Source: three-view drawing plus pictorial views. Frame: mm from the lowest corner of the part. A direction names the side the tool comes from. Give positions to 0.01 mm unless a question says otherwise; leave off trailing zeros. Write each loop counter-clockwise with the first axis right and the second up, starting at its lowest first coordinate (ties: lowest second). Pieces come first, ordered by that corner, then holes. Notation, with made-up numbers: M 48.5,28.5 L 72.5,28.5 A16 cw 72.5,57.5 Z; hole C 59.5,-28.75 d4. An arc over 180 degrees is marked long. Return JSON: item names as keys, results as strings.
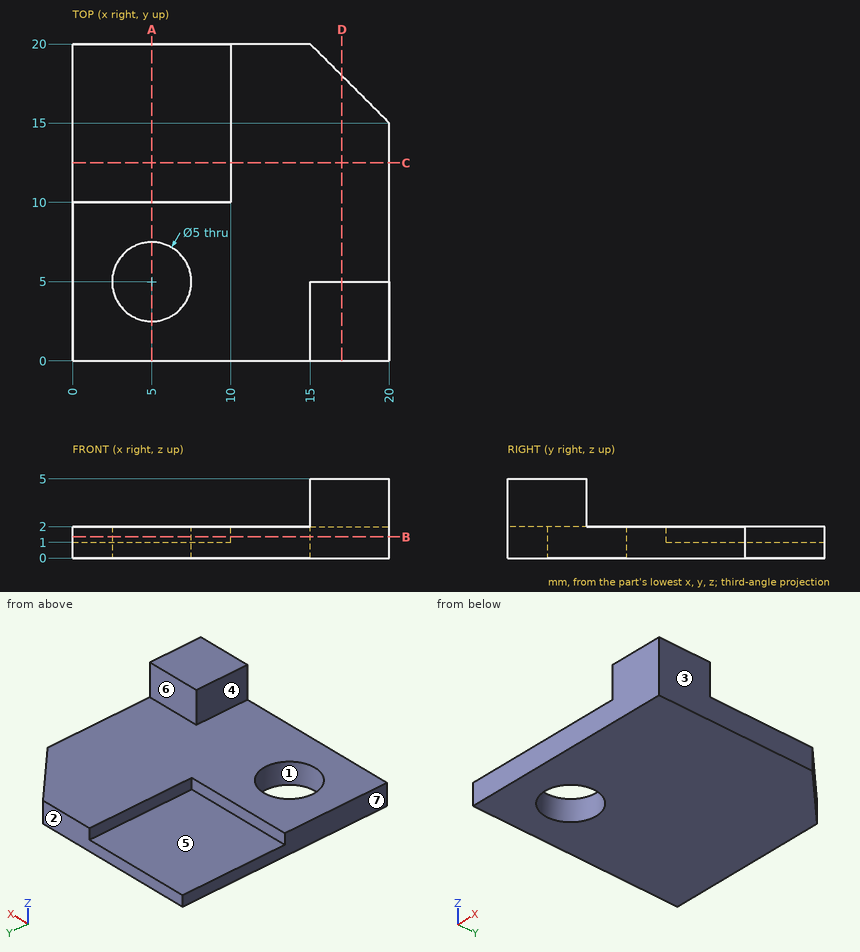
1) Cut plane D-D, the plane x = 17. Return the cut outline in (y, z).
Numbers:
{"outline": "M 0,0 L 18,0 L 18,2 L 5,2 L 5,5 L 0,5 Z"}
2) Contact query for flat-ended pins moving along their axis: pin 1 Ø4 at (x, y) = (7, 7) entering from -Z; pin 2 Ø1.5 at (x, z) = (16.5, 4) entering from +Y; pin 3 Ø0.9 at (y, z) = (2.5, 3) entering from -X; pin 4 Ø6.5 at (x, y) = (5, 5) entering from +Z. Output: stop coordinate, or through.
Numbers:
{"pin 1": "stops at z = 0", "pin 2": "stops at y = 5", "pin 3": "stops at x = 15", "pin 4": "stops at z = 2"}
3) Cut plane C-C, the plane y = 12.5. Return the cut outline in (x, z).
Numbers:
{"outline": "M 0,0 L 20,0 L 20,2 L 10,2 L 10,1 L 0,1 Z"}
4) Line query: line 1 (Y direction, x = 5, z = 1.15); line 2 (Z direction, x = 3.25, y = 14.5); line 3 (Z direction, x = 15.25, y = 16.5). Output: solid intervals per line, ascending. Write a range as [from, to].
Numbers:
{"line 1": "y = [0, 2.5], [7.5, 10]", "line 2": "z = [0, 1]", "line 3": "z = [0, 2]"}
5) Cut plane B-B, the plane z = 1.35. Return the cut outline in (x, y).
Numbers:
{"outline": "M 0,0 L 20,0 L 20,15 L 15,20 L 10,20 L 10,10 L 0,10 Z; hole C 5,5 d5"}
6) Cut plane A-A, the plane x = 5. Return the cut outline in (y, z), then the cut area to 3 significant figures.
Numbers:
{"outline": "M 0,0 L 2.5,0 L 2.5,2 L 0,2 Z; M 7.5,0 L 20,0 L 20,1 L 10,1 L 10,2 L 7.5,2 Z", "area": "20.0 mm²"}
7) Draft query along X for the marked faces 1, 2 and 3. Return one class per face: released by +X, released by -X, zero draft, split by the parting line, or undercut.
Numbers:
{"face 1": "undercut", "face 2": "zero draft", "face 3": "released by +X"}
8) Set-up query: the marked faces 4, 5, 6 and 7. Return all of +Z, -Z, +X, -X, +Y, -Y with unobstructed straight access to the full face (end or side cutting, diameter ignored); none if empty.
Numbers:
{"face 4": "+Z, -X, +Y, -Y", "face 5": "+Z, -X, +Y", "face 6": "+Z, +X, -X, +Y", "face 7": "+Z, -Z, -X, +Y, -Y"}
